from build123d import *

# Parameters (mm, degrees)
BOSS_EXTRU_1_DEPTH      = 15
CONG_1_R                = 2
ENL_V_MAT_EXTRU_1_REACH = 4
ESQUISSE2_R             = 2.5
ENL_V_MAT_EXTRU_2_REACH = 4
ESQUISSE4_R             = 2.5


with BuildPart() as part:
    # Esquisse1 → Boss.-Extru.1 (new body, symmetric)
    with BuildSketch(Plane(origin=(0, 0, 0), x_dir=(0, 0, -1), z_dir=(1, 0, 0))):
        Polygon((0, 0), (0, 140), (2, 140), (2, 2), (55, 2), (55, 0), align=None)
    extrude(amount=BOSS_EXTRU_1_DEPTH, both=True)

    # Congé1
    cong_1_edges = [part.edges().sort_by_distance(p)[0] for p in [
        (0, 0, 0),
        (0, 2, -2),
    ]]
    fillet(cong_1_edges, radius=CONG_1_R)

    # Esquisse2 → Enlèv. mat.-Extru.1 (cut, up to next)
    with BuildSketch(Plane(origin=(0, 2, 0), x_dir=(1, 0, 0), z_dir=(0, 1, 0)), mode=Mode.PRIVATE) as enl_v_mat_extru_1_sk1:
        with BuildLine():
            Line((4.25, 24.25), (4.25, 45.75))
            ThreePointArc((4.25, 45.75), (0, 50), (-4.25, 45.75))
            Line((-4.25, 45.75), (-4.25, 24.25))
            ThreePointArc((-4.25, 24.25), (0, 20), (4.25, 24.25))
        make_face()
    enl_v_mat_extru_1_tool1 = extrude(enl_v_mat_extru_1_sk1.sketch, amount=-ENL_V_MAT_EXTRU_1_REACH, mode=Mode.PRIVATE) & part.part
    add(enl_v_mat_extru_1_tool1.solids().sort_by_distance((0, 2, -35))[0], mode=Mode.SUBTRACT)
    # Esquisse2 → Enlèv. mat.-Extru.1 (cut, up to next)
    with BuildSketch(Plane(origin=(0, 2, 0), x_dir=(1, 0, 0), z_dir=(0, 1, 0)), mode=Mode.PRIVATE) as enl_v_mat_extru_1_sk2:
        with Locations((-9.5, 25)):
            Circle(ESQUISSE2_R)
    enl_v_mat_extru_1_tool2 = extrude(enl_v_mat_extru_1_sk2.sketch, amount=-ENL_V_MAT_EXTRU_1_REACH, mode=Mode.PRIVATE) & part.part
    add(enl_v_mat_extru_1_tool2.solids().sort_by_distance((-9.5, 2, -25))[0], mode=Mode.SUBTRACT)
    # Esquisse2 → Enlèv. mat.-Extru.1 (cut, up to next)
    with BuildSketch(Plane(origin=(0, 2, 0), x_dir=(1, 0, 0), z_dir=(0, 1, 0)), mode=Mode.PRIVATE) as enl_v_mat_extru_1_sk3:
        with Locations((-9.5, 45)):
            Circle(ESQUISSE2_R)
    enl_v_mat_extru_1_tool3 = extrude(enl_v_mat_extru_1_sk3.sketch, amount=-ENL_V_MAT_EXTRU_1_REACH, mode=Mode.PRIVATE) & part.part
    add(enl_v_mat_extru_1_tool3.solids().sort_by_distance((-9.5, 2, -45))[0], mode=Mode.SUBTRACT)
    # Esquisse2 → Enlèv. mat.-Extru.1 (cut, up to next)
    with BuildSketch(Plane(origin=(0, 2, 0), x_dir=(1, 0, 0), z_dir=(0, 1, 0)), mode=Mode.PRIVATE) as enl_v_mat_extru_1_sk4:
        with Locations((9.5, 45)):
            Circle(ESQUISSE2_R)
    enl_v_mat_extru_1_tool4 = extrude(enl_v_mat_extru_1_sk4.sketch, amount=-ENL_V_MAT_EXTRU_1_REACH, mode=Mode.PRIVATE) & part.part
    add(enl_v_mat_extru_1_tool4.solids().sort_by_distance((9.5, 2, -45))[0], mode=Mode.SUBTRACT)
    # Esquisse2 → Enlèv. mat.-Extru.1 (cut, up to next)
    with BuildSketch(Plane(origin=(0, 2, 0), x_dir=(1, 0, 0), z_dir=(0, 1, 0)), mode=Mode.PRIVATE) as enl_v_mat_extru_1_sk5:
        with Locations((9.5, 25)):
            Circle(ESQUISSE2_R)
    enl_v_mat_extru_1_tool5 = extrude(enl_v_mat_extru_1_sk5.sketch, amount=-ENL_V_MAT_EXTRU_1_REACH, mode=Mode.PRIVATE) & part.part
    add(enl_v_mat_extru_1_tool5.solids().sort_by_distance((9.5, 2, -25))[0], mode=Mode.SUBTRACT)

    # Esquisse4 → Enlèv. mat.-Extru.2 (cut, up to next)
    with BuildSketch(Plane(origin=(0, 0, -2), x_dir=(-1, 0, 0), z_dir=(0, 0, -1)), mode=Mode.PRIVATE) as enl_v_mat_extru_2_sk1:
        with Locations((-10, 125)):
            Circle(ESQUISSE4_R)
    enl_v_mat_extru_2_tool1 = extrude(enl_v_mat_extru_2_sk1.sketch, amount=-ENL_V_MAT_EXTRU_2_REACH, mode=Mode.PRIVATE) & part.part
    add(enl_v_mat_extru_2_tool1.solids().sort_by_distance((10, 125, -2))[0], mode=Mode.SUBTRACT)
    # Esquisse4 → Enlèv. mat.-Extru.2 (cut, up to next)
    with BuildSketch(Plane(origin=(0, 0, -2), x_dir=(-1, 0, 0), z_dir=(0, 0, -1)), mode=Mode.PRIVATE) as enl_v_mat_extru_2_sk2:
        with Locations((-10, 105)):
            Circle(ESQUISSE4_R)
    enl_v_mat_extru_2_tool2 = extrude(enl_v_mat_extru_2_sk2.sketch, amount=-ENL_V_MAT_EXTRU_2_REACH, mode=Mode.PRIVATE) & part.part
    add(enl_v_mat_extru_2_tool2.solids().sort_by_distance((10, 105, -2))[0], mode=Mode.SUBTRACT)
    # Esquisse4 → Enlèv. mat.-Extru.2 (cut, up to next)
    with BuildSketch(Plane(origin=(0, 0, -2), x_dir=(-1, 0, 0), z_dir=(0, 0, -1)), mode=Mode.PRIVATE) as enl_v_mat_extru_2_sk3:
        with Locations((-10, 85)):
            Circle(ESQUISSE4_R)
    enl_v_mat_extru_2_tool3 = extrude(enl_v_mat_extru_2_sk3.sketch, amount=-ENL_V_MAT_EXTRU_2_REACH, mode=Mode.PRIVATE) & part.part
    add(enl_v_mat_extru_2_tool3.solids().sort_by_distance((10, 85, -2))[0], mode=Mode.SUBTRACT)
    # Esquisse4 → Enlèv. mat.-Extru.2 (cut, up to next)
    with BuildSketch(Plane(origin=(0, 0, -2), x_dir=(-1, 0, 0), z_dir=(0, 0, -1)), mode=Mode.PRIVATE) as enl_v_mat_extru_2_sk4:
        with Locations((10, 115)):
            Circle(ESQUISSE4_R)
    enl_v_mat_extru_2_tool4 = extrude(enl_v_mat_extru_2_sk4.sketch, amount=-ENL_V_MAT_EXTRU_2_REACH, mode=Mode.PRIVATE) & part.part
    add(enl_v_mat_extru_2_tool4.solids().sort_by_distance((-10, 115, -2))[0], mode=Mode.SUBTRACT)
    # Esquisse4 → Enlèv. mat.-Extru.2 (cut, up to next)
    with BuildSketch(Plane(origin=(0, 0, -2), x_dir=(-1, 0, 0), z_dir=(0, 0, -1)), mode=Mode.PRIVATE) as enl_v_mat_extru_2_sk5:
        with Locations((10, 95)):
            Circle(ESQUISSE4_R)
    enl_v_mat_extru_2_tool5 = extrude(enl_v_mat_extru_2_sk5.sketch, amount=-ENL_V_MAT_EXTRU_2_REACH, mode=Mode.PRIVATE) & part.part
    add(enl_v_mat_extru_2_tool5.solids().sort_by_distance((-10, 95, -2))[0], mode=Mode.SUBTRACT)
    # Esquisse4 → Enlèv. mat.-Extru.2 (cut, up to next)
    with BuildSketch(Plane(origin=(0, 0, -2), x_dir=(-1, 0, 0), z_dir=(0, 0, -1)), mode=Mode.PRIVATE) as enl_v_mat_extru_2_sk6:
        with Locations((10, 75)):
            Circle(ESQUISSE4_R)
    enl_v_mat_extru_2_tool6 = extrude(enl_v_mat_extru_2_sk6.sketch, amount=-ENL_V_MAT_EXTRU_2_REACH, mode=Mode.PRIVATE) & part.part
    add(enl_v_mat_extru_2_tool6.solids().sort_by_distance((-10, 75, -2))[0], mode=Mode.SUBTRACT)
    # Esquisse4 → Enlèv. mat.-Extru.2 (cut, up to next)
    with BuildSketch(Plane(origin=(0, 0, -2), x_dir=(-1, 0, 0), z_dir=(0, 0, -1)), mode=Mode.PRIVATE) as enl_v_mat_extru_2_sk7:
        with BuildLine():
            Line((3.25, 130), (3.25, 70))
            ThreePointArc((3.25, 70), (0, 66.75), (-3.25, 70))
            Line((-3.25, 70), (-3.25, 130))
            ThreePointArc((-3.25, 130), (0, 133.25), (3.25, 130))
        make_face()
    enl_v_mat_extru_2_tool7 = extrude(enl_v_mat_extru_2_sk7.sketch, amount=-ENL_V_MAT_EXTRU_2_REACH, mode=Mode.PRIVATE) & part.part
    add(enl_v_mat_extru_2_tool7.solids().sort_by_distance((0, 100, -2))[0], mode=Mode.SUBTRACT)


solid = part.part
Work out the finished part from the listing and answer in its coordinate system (mm). A direction names the side the tool comes from. Round coordinates to 2 decimals unless told otherwise and drop trailing zeros. Write each loop counter-clockwise with the first axis right and the second up, starting at its lowest first coordinate (ties: lowest second). Pieces come first, ordered by that corner, then holes. Notation, with made-up numbers: (-29.5, -8.5) - (28.5, -8.5) arc R10 cw to (28.5, 4.5) - close; hole circle Ø8 at (74.5, 59.25). An arc over 180 degrees is marked (long way). Answer in a Markdown table with one row per item. Add a question column.
1. A cutting plane is placed at B-B, the plane y = 79. Determine the outline of the cut face in (x, z), and give its area (3 significant figures).
2. Find the intervals of material crossed by line 1 along Z through (x, y) = (-9.5, 0.55); line 2 along Z through (x, y) = (-9.5, 1.2); line 3 along Y through (x, z) = (-10, -1.15), in increasing order. Write a range as from..to.
3. A cutting plane is placed at D-D, the plane x = 10. Determine the outline of the cut face in (y, z), and give its area (3 significant figures).
4. Given pin 1 (1.5 mm diameter, centred on x = 10, y = 72, fed in from -Z); pin 2 (15 mm diameter, centred on x = -2, z = -32.5, fed in from +Y), each flat-ended and moving along its own axis, determine where each tip first touches the part or whether it passes through.
5. A cutting plane is placed at A-A, the plane z = -29. Determine the outline of the cut face in (x, y).
6. The mould has two halves that part along X. Classify faces 1 (the flat face through (7, 0, -29)), 2 (the cylindrical face through (0.07, 133.25, -1.01)), 3 (the cylindrical face through (10.33, 87.48, -1.01)), 4 (the flat face through (15, 70, -1)): +X half, -X half, draft (parallel to the pull), parting line (faces both ways), or undercut.
7. For faces 5 (the cylindrical face through (0, 1, -50)), 6 (the cylindrical face through (-0.07, 66.75, -1.01)), 7 (the flat face through (7, 2, -29)), determine the directions among +Z, -Z, +X, -X, +Y, -Y from which every point of the face is accessible in a straight line to the end or side of a thin tool.
8. A cutting plane is placed at C-C, the plane x = 0. Determine the outline of the cut face in (y, z).
Worked out:
| question | item | result |
|---|---|---|
| 1 | outline | (-15, -2) - (-3.25, -2) - (-3.25, 0) - (-15, 0) - close; (3.25, -2) - (15, -2) - (15, 0) - (3.25, 0) - close |
| 1 | area | 47.0 mm^2 |
| 2 | line 1 | -55..-47.5, -42.5..-27.5, -22.5..-0.62 |
| 2 | line 2 | -55..-47.5, -42.5..-27.5, -22.5..-0.17 |
| 2 | line 3 | 0.19..72.5, 77.5..92.5, 97.5..112.5, 117.5..140 |
| 3 | outline | (0, -55) - (2, -55) - (2, -47.45) - (0, -47.45) - close; (0, -42.55) - (2, -42.55) - (2, -27.45) - (0, -27.45) - close; (0, -22.55) - (2, -22.55) - (2, -4) arc R2 cw to (4, -2) - (82.5, -2) - (82.5, 0) - (2, 0) arc R2 ccw to (0, -2) - close; (87.5, -2) - (102.5, -2) - (102.5, 0) - (87.5, 0) - close; (107.5, -2) - (122.5, -2) - (122.5, 0) - (107.5, 0) - close; (127.5, -2) - (140, -2) - (140, 0) - (127.5, 0) - close |
| 3 | area | 336 mm^2 |
| 4 | pin 1 | z = -2 |
| 4 | pin 2 | y = 2 |
| 5 | outline | (-15, 0) - (-4.25, 0) - (-4.25, 2) - (-15, 2) - close; (4.25, 0) - (15, 0) - (15, 2) - (4.25, 2) - close |
| 6 | face 1 | draft |
| 6 | face 2 | undercut |
| 6 | face 3 | undercut |
| 6 | face 4 | +X half |
| 7 | face 5 | +Y, -Y |
| 7 | face 6 | +Z, -Z |
| 7 | face 7 | -Z, +X, -X, +Y |
| 8 | outline | (0, -55) - (2, -55) - (2, -50) - (0, -50) - close; (0, -20) - (2, -20) - (2, -4) arc R2 cw to (4, -2) - (66.75, -2) - (66.75, 0) - (2, 0) arc R2 ccw to (0, -2) - close; (133.25, -2) - (140, -2) - (140, 0) - (133.25, 0) - close |
